Design review of the part built by this model. Coordinates are the model's own, in mm. Round coordinates to 2 decimals unless told otherwise and drop trailing zeros. Order: outer loops, then holes, each group sorted by start corner. A loop starts at its lowest first (then second) coordinate and runs counter-clockwise, first axis right, second up. Notation, with made-up numbers: M -22,49 L 9,49 A11 cw 9,67 Z; hole C 18.5,-11 d2. An arc over 180 degrees is marked long. Use a Markdown table: item, result. Add a question column.
(1) Take a section at B-B (z = 15.25). Write out the cut boundary in (x, y).
(2) To check wall thickness, follow probe 1 along Y at (x, z) = (0, 7); probe 2 along X at (y, z) = (-19, 19); probe 3 along X at (y, z) = (19, 18.5). State the ranges of each line that lie inside material, in increasing order. Write a range as from..to.
(3) The part is to be moulded in two halves that separate along Y. For faces 1 (the face through (58.117, 17.297, 4.93)), 2 (the face through (-14.29, 64.33, 4.93)), say which applies: released by +Y, released by -Y, zero draft, split by the parting line, or undercut.
(4) For pin 1 (8.5 mm diameter, centred on x = 0, y = 58.5, fed in from +Z); pin 2 (12 mm diameter, centred on x = -10, y = -1, fed in from -Z); pin 3 (2 mm diameter, centred on y = -36, z = 10, fed in from -X); pin 4 (5 mm diameter, centred on x = 15.5, z = 10.5, fed in from -Y), all flat-tipped, find the tip position at first contact; note any pin that passes through.
(5) Take a section at A-A (x = 0). Write out the cut boundary in (y, z).
Autodesk Fusion 360 part; units mm, degrees
sketch "Boceto1" plane through (0, 0, 0) normal (0, 0, 1) x (1, 0, 0)
  circle A0 centre (0, 0) radius 65.9
  circle A1 centre (0, 58.5) radius 2.6
  circle A2 centre (0, 37.3) radius 2.6
  circle A3 centre (-18.0775, 55.6368) radius 2.6
  circle A4 centre (-11.5263, 35.4744) radius 2.6
  circle A5 centre (-34.3854, 47.3275) radius 2.6
  circle A6 centre (-21.9244, 30.1763) radius 2.6
  circle A7 centre (-47.3275, 34.3854) radius 2.6
  circle A8 centre (-30.1763, 21.9244) radius 2.6
  circle A9 centre (-55.6368, 18.0775) radius 2.6
  circle A10 centre (-35.4744, 11.5263) radius 2.6
  circle A11 centre (-58.5, 0) radius 2.6
  circle A12 centre (-37.3, 0) radius 2.6
  circle A13 centre (-55.6368, -18.0775) radius 2.6
  circle A14 centre (-35.4744, -11.5263) radius 2.6
  circle A15 centre (-47.3275, -34.3854) radius 2.6
  circle A16 centre (-30.1763, -21.9244) radius 2.6
  circle A17 centre (-34.3854, -47.3275) radius 2.6
  circle A18 centre (-21.9244, -30.1763) radius 2.6
  circle A19 centre (-18.0775, -55.6368) radius 2.6
  circle A20 centre (-11.5263, -35.4744) radius 2.6
  circle A21 centre (0, -58.5) radius 2.6
  circle A22 centre (0, -37.3) radius 2.6
  circle A23 centre (18.0775, -55.6368) radius 2.6
  circle A24 centre (11.5263, -35.4744) radius 2.6
  circle A25 centre (34.3854, -47.3275) radius 2.6
  circle A26 centre (21.9244, -30.1763) radius 2.6
  circle A27 centre (47.3275, -34.3854) radius 2.6
  circle A28 centre (30.1763, -21.9244) radius 2.6
  circle A29 centre (55.6368, -18.0775) radius 2.6
  circle A30 centre (35.4744, -11.5263) radius 2.6
  circle A31 centre (58.5, 0) radius 2.6
  circle A32 centre (37.3, 0) radius 2.6
  circle A33 centre (55.6368, 18.0775) radius 2.6
  circle A34 centre (35.4744, 11.5263) radius 2.6
  circle A35 centre (47.3275, 34.3854) radius 2.6
  circle A36 centre (30.1763, 21.9244) radius 2.6
  circle A37 centre (34.3854, 47.3275) radius 2.6
  circle A38 centre (21.9244, 30.1763) radius 2.6
  circle A39 centre (18.0775, 55.6368) radius 2.6
  circle A40 centre (11.5263, 35.4744) radius 2.6
  circle A41 centre (0, 0) radius 29.2
  circle A42 centre (0, 0) radius 6
  circle A43 centre (0, 23.3) radius 2.8
  circle A44 centre (-20.1784, 11.65) radius 2.8
  circle A45 centre (-20.1784, -11.65) radius 2.8
  circle A46 centre (0, -23.3) radius 2.8
  circle A47 centre (20.1784, -11.65) radius 2.8
  circle A48 centre (20.1784, 11.65) radius 2.8
  dimension "d2" = 5.2
  dimension "d3" = 5.2
  dimension "d6" = 360
  dimension "d13" = 58.5
  dimension "d14" = 37.3
  dimension "d16" = 131.8
  dimension "d21" = 12
  dimension "d22" = 58.4
  dimension "d23" = 5.6
  dimension "d24" = 23.3
  dimension "d26" = 360
extrude "Extruir3" add sketch "Boceto1" along normal blind 10 contours A0
extrude "Extruir4" add sketch "Boceto1" along normal blind 20 contours A41 | A43 | A44 | A45 | A46 | A47 | A48
sketch "Boceto2" plane through (0, 0, 20) normal (0, 0, 1) x (-1, 0, 0)
  circle A0 centre (0, 0) radius 6
  circle A1 centre (0, 0) radius 29.2
  circle A2 centre (-11.6857, -20.1578) radius 2.6
  circle A3 centre (11.6143, -20.199) radius 2.6
  circle A4 centre (23.3, -0.0412) radius 2.6
  circle A5 centre (11.6857, 20.1578) radius 2.6
  circle A6 centre (-11.6143, 20.199) radius 2.6
  circle A7 centre (-23.3, 0.0412) radius 2.6
  dimension "d27" = 23.3
  dimension "d29" = 360
  dimension "d32" = 5.2
extrude "Extruir5" cut sketch "Boceto2" against normal blind 20 contours A2 | A3 | A4 | A5 | A6 | A7
extrude "Extruir1" [suppressed]
extrude "Extruir2" [suppressed]
Verdict:
| question | item | result |
|---|---|---|
| 1 | outline | C 0,0 d58.4; hole C -23.3,0.04 d5.2; hole C -11.69,-20.16 d5.2; hole C -11.61,20.2 d5.2; hole C 0,0 d12; hole C 11.61,-20.2 d5.2; hole C 11.69,20.16 d5.2; hole C 23.3,-0.04 d5.2 |
| 2 | probe 1 | y = -65.9..-61.1, -55.9..-39.9, -34.7..-6, 6..34.7, 39.9..55.9, 61.1..65.9 |
| 2 | probe 2 | x = -22.17..-14.01, -9.36..9.31, 13.92..22.17 |
| 2 | probe 3 | x = -22.17..-13.92, -9.31..9.36, 14.01..22.17 |
| 3 | face 1 | undercut |
| 3 | face 2 | split by the parting line |
| 4 | pin 1 | stops at z = 10 |
| 4 | pin 2 | stops at z = 0 |
| 4 | pin 3 | stops at x = -55.84 |
| 4 | pin 4 | stops at y = -64.59 |
| 5 | outline | M -65.9,0 L -61.1,0 L -61.1,10 L -65.9,10 Z; M -55.9,0 L -39.9,0 L -39.9,10 L -55.9,10 Z; M -34.7,0 L -6,0 L -6,20 L -29.2,20 L -29.2,10 L -34.7,10 Z; M 6,0 L 34.7,0 L 34.7,10 L 29.2,10 L 29.2,20 L 6,20 Z; M 39.9,0 L 55.9,0 L 55.9,10 L 39.9,10 Z; M 61.1,0 L 65.9,0 L 65.9,10 L 61.1,10 Z |
